The model under review builds one solid part; all positions refer to its coordinate system, in mm. Face numbers are marked on the shaded views. A direction names the side the tool comes from. Coordinates: 2 decimals unless noted, no trailing zeros. Loops run counter-clockwise (first coordinate to the right, second up) from the corner with the lowest first, then second, coordinate; pieces in that order, holes last. Notation, with made-up numbers: M 82.5,-16 L 109.5,-16 A22 cw 109.5,-2 Z; hole C 11.5,53.25 d8. An arc over 180 degrees is marked long. Write item = value, one per line. Start each with the question number.
Q1. Clearance check with a flat-ended pin moving along its axis: pin 1 Ø4 at (x, z) = (-3.5, -22.5) entering from -Y. State where the tip first meets the part, or that it passes through.
Q2. We need section C-C on y = -8. Give the boundary of the cut face in (x, z).
Q3. For the marked faces 1 and 2, list the 3-axis set-ups (+Z, -Z, +X, -X, +Y, -Y) from which the entire face can be reached by the end or side of a thin tool; tool diameter is ignored.
Q4. We need section B-B on x = 0. Give the boundary of the cut face in (y, z) (3 decimals).
Q5. We need section A-A on z = 0. Give the boundary of the cut face in (x, y) (3 decimals), and give its area (3 significant figures).
Q6. Wall thickness on probe 1 along Z at (x, y) = (13, -33); probe 2 along Y at (x, z) = (-6, -1); probe 3 along Y at (x, z) = (0, 38): over which ranges is each line inside the solid? List them lowest first.
Q7. We need section D-D on x = -21.5. Give the boundary of the cut face in (y, z), and give its area (3 significant figures).
Q8. Mouldability with a two-part tool opening along Y and no side actions: class the marked faces 3, 4 and 5 as released by +Y, released by -Y, zero draft, split by the parting line, or undercut.
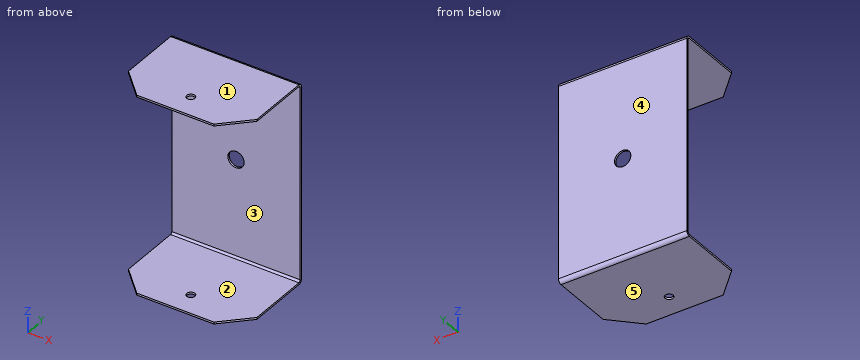
from build123d import *

# Parameters (mm, degrees)
BASE_FLANGE1_DEPTH      = 25
BASE_FLANGE1_DEPTH_BACK = 25
SKETCH6_R               = 1.5875
CUT_EXTRUDE1_DEPTH      = 89.786969755
SKETCH7_R               = 3.175
CUT_EXTRUDE2_DEPTH      = 10
CHAMFER1_SIZE           = 10


# Sheet-metal steps are written as plain solids
with BuildPart() as part:
    # Sketch1 → Base-Flange1 (new, two sides: drawn at the far end of the back side and taken through both)
    with BuildSketch(Plane(origin=(0, 0, 0), x_dir=(0, 0, -1), z_dir=(1, 0, 0)).offset(-BASE_FLANGE1_DEPTH_BACK)):
        with BuildLine():
            Line((-38.1, -35), (-38.1, -0.7366))
            ThreePointArc((-38.1, -0.7366), (-37.884254855, -0.215745145), (-37.3634, 0))
            Line((-37.3634, 0), (37.3634, 0))
            ThreePointArc((37.3634, 0), (37.884254855, -0.215745145), (38.1, -0.7366))
            Line((38.1, -0.7366), (38.1, -35))
            Line((38.1, -35), (38.8366, -35))
            Line((38.8366, -35), (38.8366, -0.7366))
            ThreePointArc((38.8366, -0.7366), (38.40510971, 0.30510971), (37.3634, 0.7366))
            Line((37.3634, 0.7366), (-37.3634, 0.7366))
            ThreePointArc((-37.3634, 0.7366), (-38.40510971, 0.30510971), (-38.8366, -0.7366))
            Line((-38.8366, -0.7366), (-38.8366, -35))
            Line((-38.8366, -35), (-38.1, -35))
        make_face()
    extrude(amount=BASE_FLANGE1_DEPTH + BASE_FLANGE1_DEPTH_BACK)

    # Sketch6 → Cut-Extrude1 (cut, through all)
    with BuildSketch(Plane(origin=(0, 0, -38.8366), x_dir=(-1, 0, 0), z_dir=(0, 0, -1))):
        with Locations(Location((0, -26.05331339, 0), (0, 0, 90))):
            Circle(SKETCH6_R)
    extrude(amount=-CUT_EXTRUDE1_DEPTH, mode=Mode.SUBTRACT)

    # Sketch7 → Cut-Extrude2 (cut)
    with BuildSketch(Plane(origin=(0, 0.7366, 0), x_dir=(1, 0, 0), z_dir=(0, 1, 0))):
        with Locations(Location((0, 0, 0), (0, 0, 270))):
            Circle(SKETCH7_R)
    extrude(amount=-CUT_EXTRUDE2_DEPTH, mode=Mode.SUBTRACT)

    # Chamfer1
    chamfer1_edges = [part.edges().sort_by_distance(p)[0] for p in [
        (25, -35, -38.4683),
        (-25, -35, -38.4683),
        (-25, -35, 38.4683),
        (25, -35, 38.4683),
    ]]
    chamfer(chamfer1_edges, length=CHAMFER1_SIZE)


solid = part.part
Returned:
q1.pin_1 = 0
q2.outline = M -25,-38.84 L 25,-38.84 L 25,-38.1 L -25,-38.1 Z; M -25,38.1 L 25,38.1 L 25,38.84 L -25,38.84 Z
q3.face_1 = +Z, +X, -X, +Y, -Y
q3.face_2 = +X, -X, -Y
q4.outline = M -35,-38.837 L -27.641,-38.837 L -27.641,-38.1 L -35,-38.1 Z; M -35,38.1 L -27.641,38.1 L -27.641,38.837 L -35,38.837 Z; M -24.466,-38.837 L -0.737,-38.837 A1.473 ccw 0.737,-37.363 L 0.737,-3.175 L 0,-3.175 L 0,-37.363 A0.737 cw -0.737,-38.1 L -24.466,-38.1 Z; M -24.466,38.1 L -0.737,38.1 A0.737 cw 0,37.363 L 0,3.175 L 0.737,3.175 L 0.737,37.363 A1.473 ccw -0.737,38.837 L -24.466,38.837 Z
q5.outline = M -25,0 L -3.175,0 L -3.175,0.737 L -25,0.737 Z; M 3.175,0 L 25,0 L 25,0.737 L 3.175,0.737 Z
q5.area = 32.2 mm^2
q6.probe_1 = -38.84 to -38.1, 38.1 to 38.84
q6.probe_2 = 0 to 0.74
q6.probe_3 = -0.37 to 0.59
q7.outline = M -28.5,-38.84 L -0.74,-38.84 A1.47 ccw 0.74,-37.36 L 0.74,37.36 A1.47 ccw -0.74,38.84 L -28.5,38.84 L -28.5,38.1 L -0.74,38.1 A0.74 cw 0,37.36 L 0,-37.36 A0.74 cw -0.74,-38.1 L -28.5,-38.1 Z
q7.area = 98.5 mm^2
q8.face_3 = released by -Y
q8.face_4 = released by +Y
q8.face_5 = zero draft
